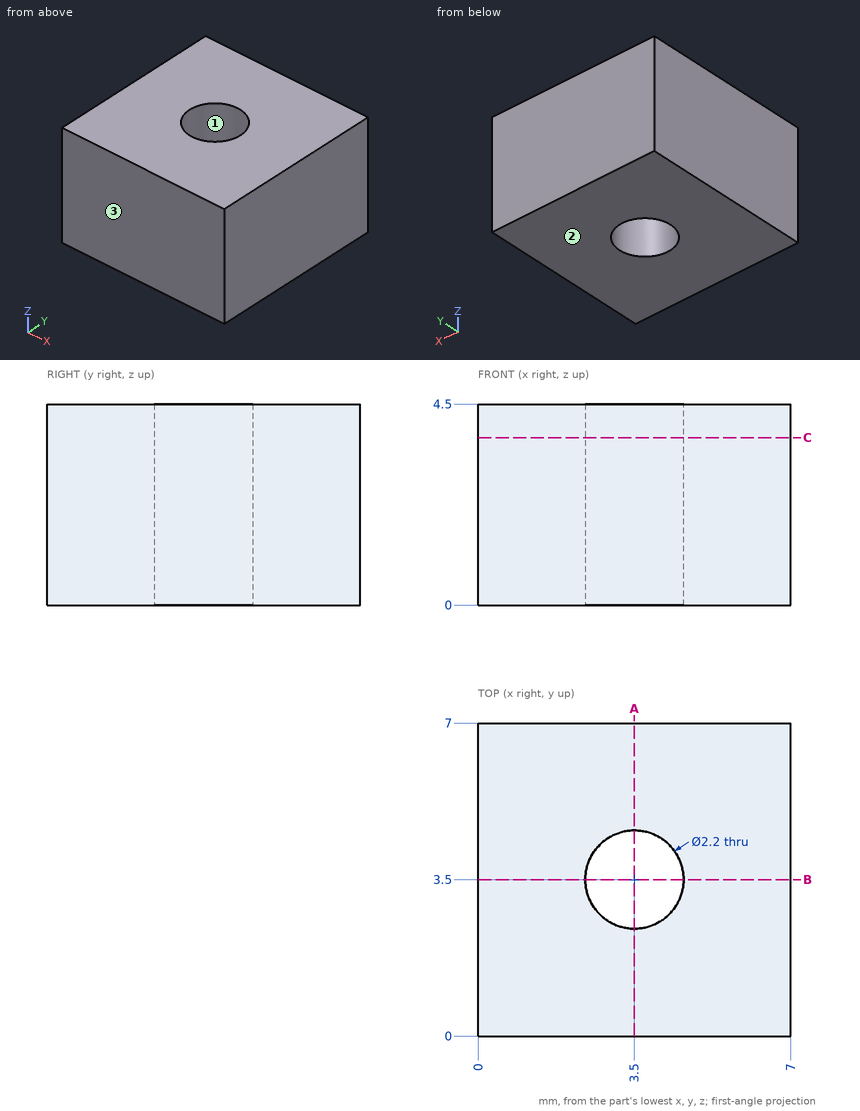
The drawing under review shows one solid part. Ordinate dimensions are in mm from its lowest x, y, z. Round coordinates to 2 decimals unless told otherwise and drop trailing zeros. Order: outer loops, then holes, each group sorted by start corner. A loop starts at its lowest first (then second) coordinate and runs counter-clockwise, first axis right, second up. Notation, with made-up numbers: M 76.5,70 L 107.5,70 A22 ccw 107.5,95 Z; hole C 31.25,-10 d9. An arc over 180 degrees is marked long. Answer as CSV lines item,"result". Start each with the question number.
1) Add section A-A (x = 3.5). Give the boundary of the cut face in (y, z), then the cut area to 3 significant figures.
2) Wall thickness on line 1 along X through (y, z) = (3.5, 2.15); line 2 along Y through (x, z) = (3, 0.55): over which ranges is each line inside the solid? List them lowest first. Write a range as [from, to].
3) Add section C-C (z = 3.75). Give the boundary of the cut face in (x, y), then the cut area to 3 significant figures.
4) The part is to be moulded in two halves that separate along Y. For the marked faces 1, 2 and 3, say which applies: +Y half, -Y half, draft (parallel to the pull), parting line (faces both ways), or undercut.
Resolved:
1,outline,"M 0,0 L 2.4,0 L 2.4,4.5 L 0,4.5 Z; M 4.6,0 L 7,0 L 7,4.5 L 4.6,4.5 Z"
1,area,"21.6 mm^2"
2,line 1,"[0, 2.4], [4.6, 7]"
2,line 2,"[0, 2.52], [4.48, 7]"
3,outline,"M 0,0 L 7,0 L 7,7 L 0,7 Z; hole C 3.5,3.5 d2.2"
3,area,"45.2 mm^2"
4,face 1,"undercut"
4,face 2,"draft"
4,face 3,"-Y half"
